Drawing for the job (mm, zero at the part's lowest x, y, z). Coordinates: 2 decimals unless noted, no trailing zeros. Write each loop counter-clockwise with the first axis right and the second up, starting at its lowest first coordinate (ties: lowest second). Pieces come first, ordered by that corner, then holes.
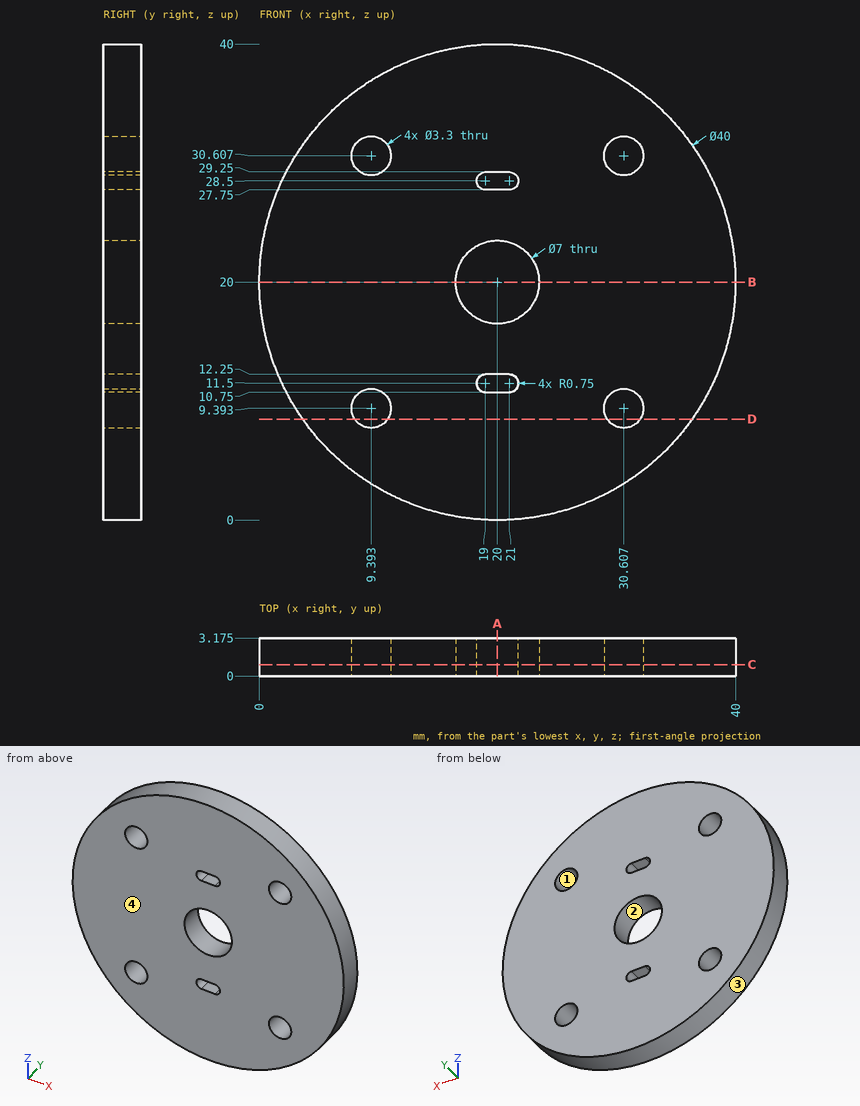
Item 1: Two-plate mould, pull along X, no slides. Class the marked faces 1, 2, 3 and 4: +X half, -X half, draft (parallel to the pull), parting line (faces both ways), or undercut.
Item 2: Saw through at B-B, the plane z = 20. Write the cut outline in (x, y) (1 decimal).
Item 3: Saw through at C-C, the plane y = 0.95. Write the cut outline in (x, z), and give its area (3 significant figures).
Item 4: Saw through at A-A, the plane x = 20. State how many separate pieces and enclosed holes the cut face has.
Item 5: Saw through at D-D, the plane z = 8.5. Write the cut outline in (x, y) (1 decimal).
Item 6: Flat gauge pins, fed straight in: pin 1 Ø2.5 at (x, z) = (30.61, 30.61) entering from -Y (1 decimal); pin 2 Ø0.6 at (x, y) = (20.5, 1.5) entering from -Z. Where does each tip first touch, or does it go through?
Item 7: Wall check: line 1 along X through (y, z) = (2.7, 8) (1 decimal); line 2 along X through (y, z) = (0.65, 31) (1 decimal); line 3 along Z through (x, y) = (10, 1.35). Give the ranges that are in metal, low to high.
Working result:
1. face 1: undercut
1. face 2: undercut
1. face 3: parting line
1. face 4: draft
2. outline: (0, 0) - (16.5, 0) - (16.5, 3.2) - (0, 3.2) - close; (23.5, 0) - (40, 0) - (40, 3.2) - (23.5, 3.2) - close
3. outline: circle Ø40 at (20, 20); hole circle Ø3.3 at (9.39, 9.39); hole circle Ø3.3 at (9.39, 30.61); hole circle Ø7 at (20, 20); hole (19, 10.75) - (21, 10.75) arc R0.75 ccw to (21, 12.25) - (19, 12.25) arc R0.75 ccw to start; hole (19, 27.75) - (21, 27.75) arc R0.75 ccw to (21, 29.25) - (19, 29.25) arc R0.75 ccw to start; hole circle Ø3.3 at (30.61, 9.39); hole circle Ø3.3 at (30.61, 30.61)
3. area: 1,170 mm2
4. separate pieces: 4
4. enclosed holes: 0
5. outline: (3.6, 0) - (8, 0) - (8, 3.2) - (3.6, 3.2) - close; (10.8, 0) - (29.2, 0) - (29.2, 3.2) - (10.8, 3.2) - close; (32, 0) - (36.4, 0) - (36.4, 3.2) - (32, 3.2) - close
6. pin 1: passes through
6. pin 2: stops at z = 0
7. line 1: x = 4 to 8.5, 10.3 to 29.7, 31.5 to 36
7. line 2: x = 3.3 to 7.8, 11 to 29, 32.2 to 36.7
7. line 3: z = 2.68 to 7.86, 10.93 to 29.07, 32.14 to 37.32
